The drawing under review shows one solid part. Ordinate dimensions are in mm from its lowest x, y, z. A direction names the side the tool comes from. Round coordinates to 2 decimals unless told otherwise and drop trailing zeros. Write each loop counter-clockwise with the first axis right and the second up, starting at its lowest first coordinate (ties: lowest second). Pieces come first, ordered by that corner, then holes. Notation, with made-up numbers: (-11, 37.5) -> (30, 37.5) arc R20 ccw to (30, 56.5) -> close; hole circle Ø11 at (27, -6.75). An arc over 180 degrees is marked (long way). Use CSV: the item, a comma, the result in double quotes. Start each with the question number.
1) Take a section at D-D, the plane z = 5. Give the boundary of the cut face in (x, y), then the cut area to 3 significant figures.
2) Take a section at C-C, the plane z = 20.5. Give the boundary of the cut face in (x, y), then the cut area to 3 significant figures.
3) For pin 1 Ø4 at (y, z) = (19.5, 20.5) entering from -X; pin 2 Ø5 at (x, z) = (40, 6) entering from -Y; pin 3 Ø3 at (x, y) = (31.5, 2.5) entering from -Z; pin 4 Ø2 at (x, z) = (36, 5) entering from +Y, all flat-tipped, find the tip position at first contact; note any pin that passes through.
4) Mouldability with a two-part tool opening along X and no side actions: class the marked faces 1, 2 and 3 as released by +X, released by -X, zero draft, split by the parting line, or undercut.
5) Machinability: for the marked faces 4, 5, 6, 7 and 8, which of the approach directions +Z, -Z, +X, -X, +Y, -Y give a long, thin tool a straight path to every point of the face, cutting with its end or side? Answer none if there is none.
6) Take a section at A-A, the plane y = 15.75. Give the boundary of the cut face in (x, z).
7) Wall thickness on probe 1 along Z at (x, y) = (36, 7.25); probe 2 along Y at (x, z) = (6, 19.5); probe 3 along X at (y, z) = (12, 8.75): over which ranges is each line inside the solid? List them lowest first. Write a range as [from, to].
8) Take a section at B-B, the plane x = 36. Give the boundary of the cut face in (y, z), then the cut area to 3 significant figures.
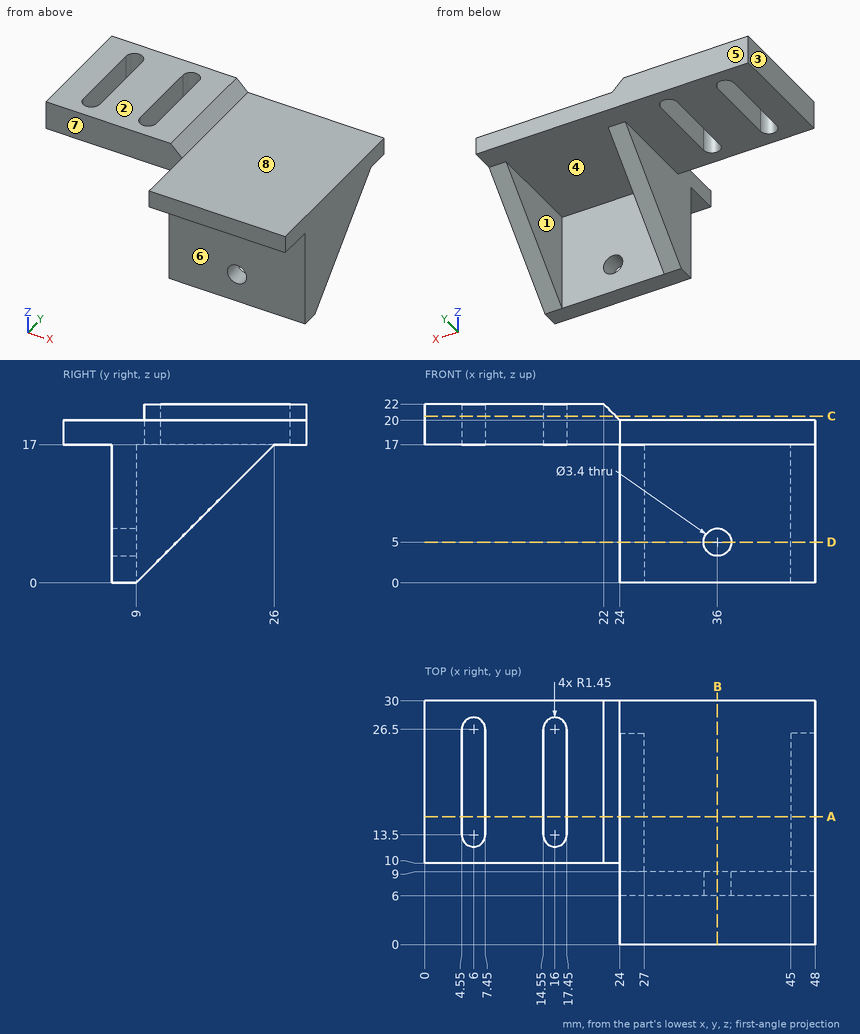
Values found:
1,outline,"(24, 6) -> (34.3, 6) -> (34.3, 9) -> (27, 9) -> (27, 14) -> (24, 14) -> close; (37.7, 6) -> (48, 6) -> (48, 14) -> (45, 14) -> (45, 9) -> (37.7, 9) -> close"
1,area,"91.8 mm²"
2,outline,"(0, 10) -> (23.5, 10) -> (23.5, 30) -> (0, 30) -> close; hole (4.55, 13.5) arc R1.45 ccw to (7.45, 13.5) -> (7.45, 26.5) arc R1.45 ccw to (4.55, 26.5) -> close; hole (14.55, 13.5) arc R1.45 ccw to (17.45, 13.5) -> (17.45, 26.5) arc R1.45 ccw to (14.55, 26.5) -> close"
2,area,"381 mm²"
3,pin 1,"x = 0"
3,pin 2,"y = 6"
3,pin 3,"z = 17"
3,pin 4,"through"
4,face 1,"undercut"
4,face 2,"zero draft"
4,face 3,"released by -X"
5,face 4,"-Z, +Y"
5,face 5,"+Z, -Z, +X, -X, +Y"
5,face 6,"-Z, +X, -X, -Y"
5,face 7,"+Z, -Z, -X, -Y"
5,face 8,"+Z, +X, +Y, -Y"
6,outline,"(0, 17) -> (4.55, 17) -> (4.55, 22) -> (0, 22) -> close; (7.45, 17) -> (14.55, 17) -> (14.55, 22) -> (7.45, 22) -> close; (17.45, 17) -> (24, 17) -> (24, 6.75) -> (27, 6.75) -> (27, 17) -> (45, 17) -> (45, 6.75) -> (48, 6.75) -> (48, 20) -> (24, 20) -> (22, 22) -> (17.45, 22) -> close"
7,probe 1,"[0, 3.3], [6.7, 20]"
7,probe 2,"[10, 12.05], [27.95, 30]"
7,probe 3,"[24, 27], [45, 48]"
8,outline,"(0, 17) -> (6, 17) -> (6, 6.7) -> (9, 6.7) -> (9, 17) -> (30, 17) -> (30, 20) -> (0, 20) -> close; (6, 0) -> (9, 0) -> (9, 3.3) -> (6, 3.3) -> close"
8,area,"131 mm²"
